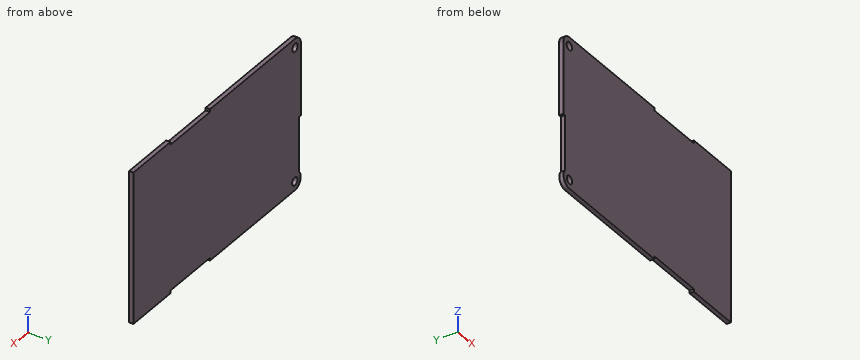
```python
from build123d import *

# Parameters (mm, degrees)
SKETCH1_R           = 1.6
BOSS_EXTRUDE1_DEPTH = 1.7


with BuildPart() as part:
    # Sketch1 → Boss-Extrude1 (new body)
    with BuildSketch(Plane(origin=(0, 0, 0), x_dir=(1, 0, 0), z_dir=(0, 1, 0))):
        with BuildLine():
            ThreePointArc((0, 3.5), (1.025126266, 1.025126266), (3.5, 0))
            Line((3.5, 0), (54, 0))
            Line((54, 0), (54, 1.1))
            Line((54, 1.1), (77.5, 1.1))
            Line((77.5, 1.1), (77.5, 0))
            Line((77.5, 0), (99.5, 0))
            Line((99.5, 0), (99.5, 59.5))
            Line((99.5, 59.5), (77.5, 59.5))
            Line((77.5, 59.5), (77.5, 58.4))
            Line((77.5, 58.4), (54, 58.4))
            Line((54, 58.4), (54, 59.5))
            Line((54, 59.5), (3.6, 59.5))
            ThreePointArc((3.6, 59.5), (0.402285022, 57.422891043), (1, 53.656925097))
            Line((1, 53.656925097), (1, 32))
            Line((1, 32), (0, 32))
            Line((0, 32), (0, 3.5))
        make_face()
        with Locations(Location((3.5, 3.5, 0), (0, 0, 270))):
            Circle(SKETCH1_R, mode=Mode.SUBTRACT)
        with Locations(Location((3.6, 56, 0), (0, 0, 270))):
            Circle(SKETCH1_R, mode=Mode.SUBTRACT)
    extrude(amount=BOSS_EXTRUDE1_DEPTH)


solid = part.part
```
Design review of the part built by this model. Coordinates are the model's own, in mm. Round coordinates to 2 decimals unless told otherwise and drop trailing zeros. Order: outer loops, then holes, each group sorted by start corner. A loop starts at its lowest first (then second) coordinate and runs counter-clockwise, first axis right, second up. Notation, with made-up numbers: M 34,-2.5 L 78,-2.5 A21 cw 78,29.5 Z; hole C -25,9 d7. An arc over 180 degrees is marked long. Put each result on its own line as item: value.
Q1. Consider section B-B (y = 1.3). State the section outline as (x, z) points, and give its area (3 significant figures).
Reported:
outline: M 0,-32 L 1,-32 L 1,-53.66 A3.5 ccw 3.6,-59.5 L 54,-59.5 L 54,-58.4 L 77.5,-58.4 L 77.5,-59.5 L 99.5,-59.5 L 99.5,0 L 77.5,0 L 77.5,-1.1 L 54,-1.1 L 54,0 L 3.5,0 A3.5 ccw 0,-3.5 Z; hole C 3.5,-3.5 d3.2; hole C 3.6,-56 d3.2
area: 5,820 mm²
Q2. To check wall thickness, follow line 1 (X direction, y = 0.95, z = -56); line 2 (Z direction, x = 58.5, y = 1.15); line 3 (X direction, y = 0.4, z = -55). State the ranges of each line that lie inside material, in increasing order.
Reported:
line 1: 0.1 to 2, 5.2 to 99.5
line 2: -58.4 to -1.1
line 3: 0.25 to 2.35, 4.85 to 99.5
Q3. Consider section A-A (z = -56). State the section outline as (x, y) points.
Reported:
outline: M 0.1,0 L 2,0 L 2,1.7 L 0.1,1.7 Z; M 5.2,0 L 99.5,0 L 99.5,1.7 L 5.2,1.7 Z
Q4. Insertion check: pin 1 Ø0.8 at (x, y) = (0.5, 0.5) entering from -Z; pin 2 Ø0.5 at (x, y) = (70, 1) entering from -Z; pin 3 Ø0.5 at (x, y) = (65, 0.5) entering from +Z. Each pin has a flat end and moves straight along its axis. Give the tip position at first contact, or say it passes through.
Reported:
pin 1: z = -58.23
pin 2: z = -58.4
pin 3: z = -1.1
